from build123d import *

# Parameters (mm, degrees)
SKETCH_1_W          = 7
SKETCH_1_H          = 8.9
EXTRUDE_1_DEPTH     = 21.5
FILLET_1_R          = 1
SKETCH_6_R          = 1.65
CUT_EXTRUDE_2_DEPTH = 10
SKETCH_7_R          = 1.65
CUT_EXTRUDE_3_DEPTH = 10
FILLET_3_R          = 3


with BuildPart() as part:
    # 草图1 → 凸台-拉伸1 (new body)
    with BuildSketch(Plane.XY):
        with Locations((3.5, 4.45)):
            Rectangle(SKETCH_1_W, SKETCH_1_H)
    extrude(amount=EXTRUDE_1_DEPTH)

    # 圆角1
    fillet_1_edges = [part.edges().sort_by_distance(p)[0] for p in [
        (3.5, 8.9, 21.5),
        (3.5, 8.9, 0),
        (7, 4.45, 0),
        (3.5, 0, 0),
        (0, 4.45, 0),
        (3.5, 0, 21.5),
        (0, 8.9, 10.75),
        (7, 8.9, 10.75),
        (7, 0, 10.75),
        (0, 0, 10.75),
    ]]
    fillet(fillet_1_edges, radius=FILLET_1_R)

    # 草图6 → 切除-拉伸2 (cut)
    with BuildSketch(Plane.ZY):
        with Locations((3.5, 4.45)):
            Circle(SKETCH_6_R)
        with Locations((13, 4.45)):
            Circle(SKETCH_6_R)
    extrude(amount=-CUT_EXTRUDE_2_DEPTH, mode=Mode.SUBTRACT)

    # 草图7 → 切除-拉伸3 (cut)
    with BuildSketch(Plane(origin=(0, 8.9, 0), x_dir=(1, 0, 0), z_dir=(0, 1, 0))):
        with Locations(Location((3.5, -8, 0), (0, 0, 270))):
            Circle(SKETCH_7_R)
        with Locations(Location((3.5, -18, 0), (0, 0, 270))):
            Circle(SKETCH_7_R)
    extrude(amount=-CUT_EXTRUDE_3_DEPTH, mode=Mode.SUBTRACT)

    # 圆角3
    # the kernel refuses this fillet: 3 mm, written as the material it takes off along each edge
    with BuildSketch(Plane(origin=(3, 0, 18.5), x_dir=(0, 0, 1), z_dir=(1, 0, 0))) as fillet_3_piece_1:
        with BuildLine():
            CenterArc((2, -1), 1, 0, 90)
            Line((3, -1), (3, 0))
            Line((3, 0), (2, 0))
        make_face()
    revolve(axis=Axis((3, 0, 18.5), (0, -1, 0)), revolution_arc=90, mode=Mode.SUBTRACT)
    with BuildSketch(Plane(origin=(3, 8.9, 18.5), x_dir=(-1, 0, 0), z_dir=(0, 0, -1))) as fillet_3_piece_2:
        with BuildLine():
            CenterArc((2, -1), 1, 0, 90)
            Line((3, -1), (3, 0))
            Line((3, 0), (2, 0))
        make_face()
    revolve(axis=Axis((3, 8.9, 18.5), (0, 1, 0)), revolution_arc=90, mode=Mode.SUBTRACT)
    with BuildSketch(Plane(origin=(0, 8.9, 21.5), x_dir=(0, 0, -1), z_dir=(0, -1, 0))) as fillet_3_piece_3:
        with BuildLine():
            CenterArc((FILLET_3_R, FILLET_3_R), FILLET_3_R, 180, 90)
            Line((0, FILLET_3_R), (0, 0))
            Line((0, 0), (FILLET_3_R, 0))
        make_face()
    extrude(amount=8.9, mode=Mode.SUBTRACT)


solid = part.part
Here's how the part is built. I have some questions about the finished solid (model axes, mm). Coordinates: 2 decimals unless noted, no trailing zeros. Write each loop counter-clockwise with the first axis right and the second up, starting at its lowest first coordinate (ties: lowest second). Pieces come first, ordered by that corner, then holes.
Item 1: I want a section at D-D on y = 1.5. Write out the boundary of the cut face in (x, z).
Item 2: If we mould it in two halves opening along Z, with no side actions, what happens to faces 1 (the flat face through (3, 0, 11)), 2 (the cylindrical face through (0.285, 4.498, 0.301)), 3 (the cylindrical face through (3.996, 4.512, 19.574))? For each: +Z half, -Z half, draft (parallel to the pull), parting line (faces both ways), or undercut.
Item 3: I want a section at B-B on z = 8. Write out the boundary of the cut face in (x, y).
Item 4: I want a section at C-C on x = 5.75. Write out the boundary of the cut face in (y, z).
Item 5: Will these pins go through, and if not, where does the flat tip stop? pin 1 (2 mm diameter, centred on x = 3.5, z = 8, fed in from +Y); pin 2 (1.5 mm diameter, centred on x = 1.5, y = 5.5, fed in from +Z).
Item 6: I want a section at A-A on x = 3.5. Write out the boundary of the cut face in (y, z).
Item 7: If I drill on line 1 (X direction, y = 4.25, z = 8); line 2 (Z direction, x = 4, y = 1.5); line 3 (Z direction, x = 2.75, y = 4.5), over which ranges is the centre line in solid material (lowest first)?
Findings below:
1. outline: (0, 1) arc R1 ccw to (1, 0) - (6, 0) arc R1 ccw to (7, 1) - (7, 21.5) - (3, 21.5) arc R3 ccw to (0, 18.5) - close; hole circle Ø3.3 at (3.5, 8); hole circle Ø3.3 at (3.5, 18)
2. face 1: draft
2. face 2: -Z half
2. face 3: undercut
3. outline: (0, 1) arc R1 ccw to (1, 0) - (1.85, 0) - (1.85, 8.9) - (1, 8.9) arc R1 ccw to (0, 7.9) - close; (5.15, 0) - (6, 0) arc R1 ccw to (7, 1) - (7, 7.9) arc R1 ccw to (6, 8.9) - (5.15, 8.9) - close
4. outline: (0, 1) arc R1 ccw to (1, 0) - (7.9, 0) arc R1 ccw to (8.9, 1) - (8.9, 20.5) arc R1 ccw to (7.9, 21.5) - (1, 21.5) arc R1 ccw to (0, 20.5) - close; hole circle Ø3.3 at (4.45, 3.5); hole circle Ø3.3 at (4.45, 13)
5. pin 1: passes through
5. pin 2: stops at z = 21.4
6. outline: (0, 1) arc R1 ccw to (1, 0) - (7.9, 0) arc R1 ccw to (8.9, 1) - (8.9, 6.35) - (0, 6.35) - close; (0, 9.65) - (8.9, 9.65) - (8.9, 16.35) - (0, 16.35) - close; (0, 19.65) - (8.9, 19.65) - (8.9, 20.5) arc R1 ccw to (7.9, 21.5) - (1, 21.5) arc R1 ccw to (0, 20.5) - close; hole circle Ø3.3 at (4.45, 3.5); hole circle Ø3.3 at (4.45, 13)
7. line 1: x = 0 to 1.85, 5.15 to 7
7. line 2: z = 0 to 6.43, 9.57 to 16.43, 19.57 to 21.5
7. line 3: z = 0 to 1.85, 5.15 to 6.53, 9.47 to 11.35, 14.65 to 16.53, 19.47 to 21.49
